Geometry: see drawing. Coordinates: mm, zero at the bounding-box minimum. A direction names the side the tool comes from. Give positions to 0.01 mm unless a question says otherwise; leave off trailing zeros. Order: outer loops, then holes, each group sorted by start corner. A loop starts at its lowest first (then second) coordinate and runs counter-clockwise, first axis right, second up. Notation, with made-up numbers: (14.25, -9.75) - (22.25, -9.75) arc R23 cw to (22.25, 12.25) - close; hole circle Ø8 at (82, 73). An arc over 180 degrees is marked (long way). Write item = value, one per line. Start each with the question number.
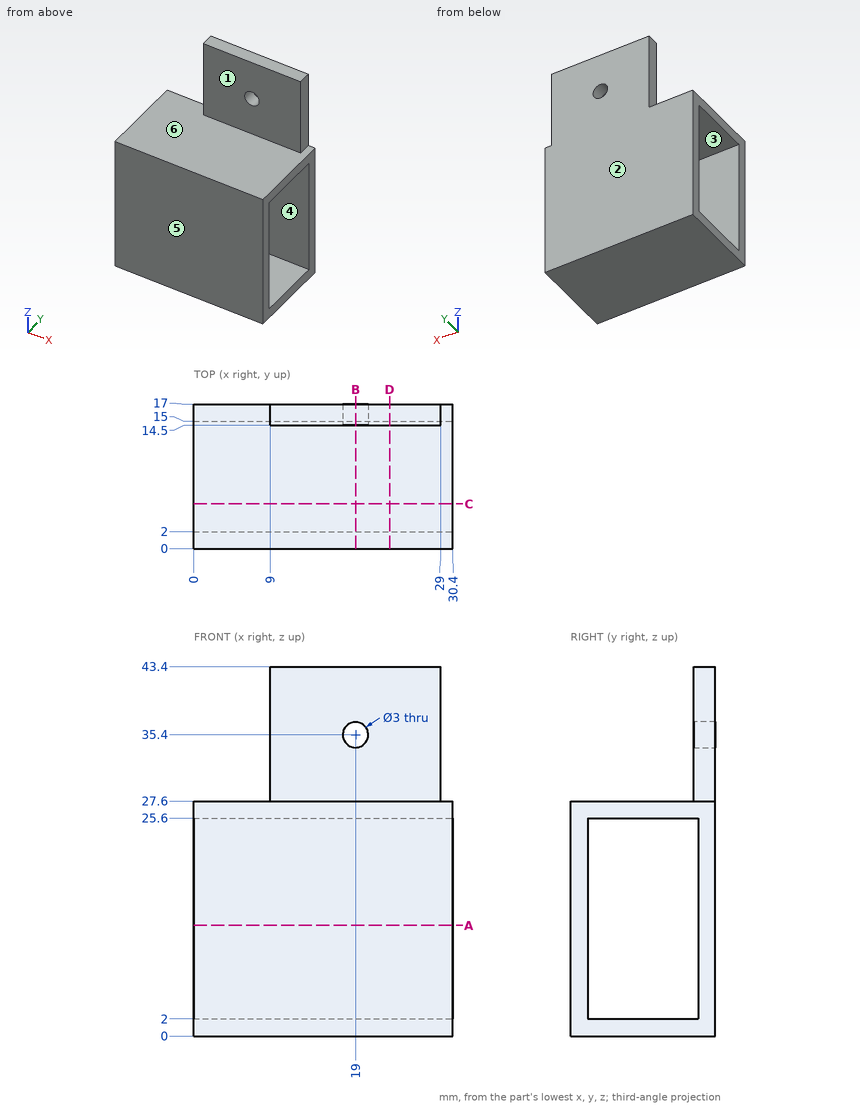
Q1. Pull-direction query (Y, two-part tool) for the marked faces 4, 5 and 6; classes: +Y half, -Y half, draft (parallel to the pull), parting line (faces both ways), or undercut.
Q2. Set-up query: the marked faces 1, 2 and 3. Return all of +Z, -Z, +X, -X, +Y, -Y with unobstructed straight access to the full face (end or side cutting, diameter ignored); none if empty.
Q3. Section D-D, the plane x = 23. Return the cut outline in (y, z).
Q4. Section C-C, the plane y = 5.25. Return the cut outline in (x, z), then the cut area to 3 significant figures.
Q5. Section A-A, the plane z = 13. Return the cut outline in (x, y).
Q6. Section B-B, the plane x = 19. Return the cut outline in (y, z), then the cut area to 3 significant figures.
Q7. Contact query for flat-ended pins moving along their axis: pin 1 (6.5 mm diameter, centred on x = 14, y = 8.5, fed in from -Z); pin 2 (2 mm diameter, centred on y = 16.5, z = 32.5, fed in from +X); pin 3 (8 mm diameter, centred on x = 20, z = 37, fed in from -Y); pin 4 (1.2 mm diameter, centred on y = 16, z = 34, fed in from -X). Output: stop coordinate, or through.
Q8. Material intervals for line 1 along Z through (x, y) = (18.5, 4); line 2 along Y through (x, z) = (6, 13); line 3 along X through (y, z) = (15.85, 35.4), sorted ascending. Write a range as from..to.
The answers:
q1.face_4 = undercut
q1.face_5 = -Y half
q1.face_6 = draft
q2.face_1 = +Z, +X, -X, -Y
q2.face_2 = +Z, -Z, +X, -X, +Y
q2.face_3 = +X, -X
q3.outline = (0, 0) - (17, 0) - (17, 43.4) - (14.5, 43.4) - (14.5, 27.6) - (0, 27.6) - close; hole (2, 2) - (15, 2) - (15, 25.6) - (2, 25.6) - close
q4.outline = (0, 0) - (30.4, 0) - (30.4, 2) - (0, 2) - close; (0, 25.6) - (30.4, 25.6) - (30.4, 27.6) - (0, 27.6) - close
q4.area = 122 mm²
q5.outline = (0, 0) - (30.4, 0) - (30.4, 2) - (0, 2) - close; (0, 15) - (30.4, 15) - (30.4, 17) - (0, 17) - close
q6.outline = (0, 0) - (17, 0) - (17, 33.9) - (14.5, 33.9) - (14.5, 27.6) - (0, 27.6) - close; (14.5, 36.9) - (17, 36.9) - (17, 43.4) - (14.5, 43.4) - close; hole (2, 2) - (15, 2) - (15, 25.6) - (2, 25.6) - close
q6.area = 194 mm²
q7.pin_1 = 0
q7.pin_2 = 29
q7.pin_3 = 14.5
q7.pin_4 = 9
q8.line_1 = 0..2, 25.6..27.6
q8.line_2 = 0..2, 15..17
q8.line_3 = 9..17.5, 20.5..29
